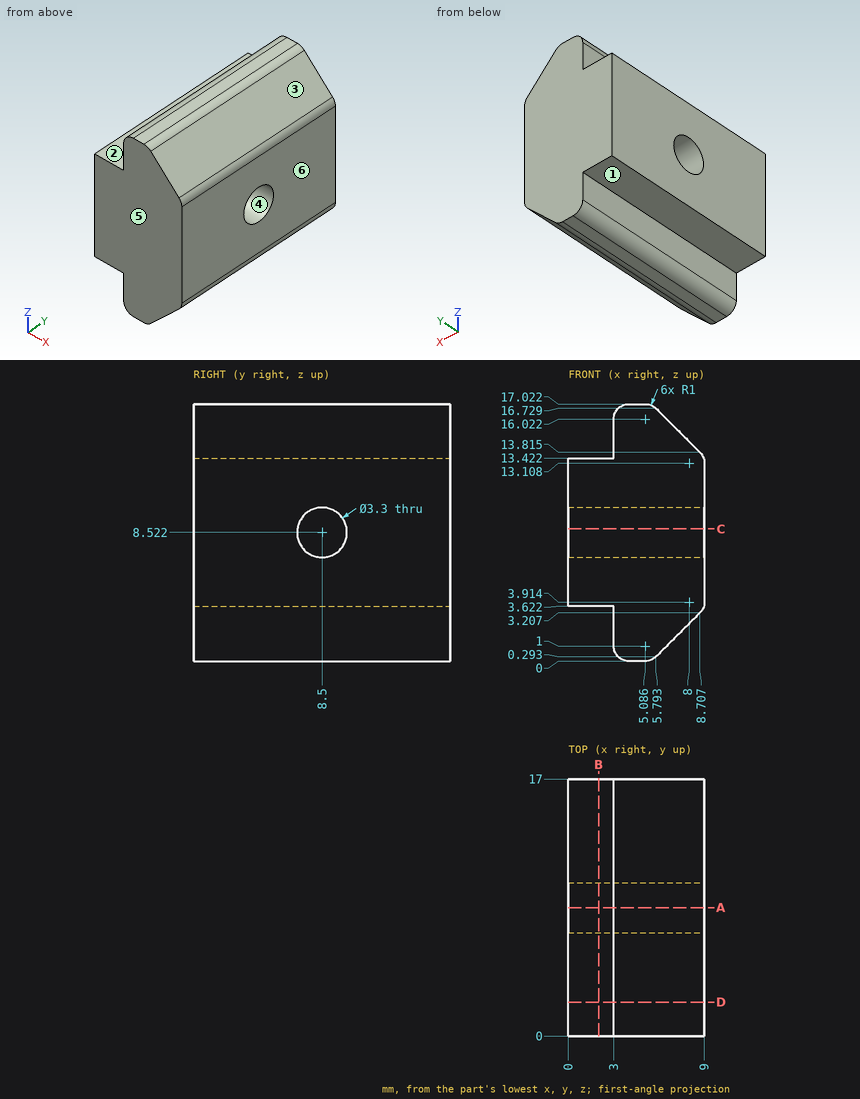
Here's the drawing with two shaded views (mm, measured from the low corner). I have some questions. A direction names the side the tool comes from. Coordinates: 2 decimals unless noted, no trailing zeros. Write each loop counter-clockwise with the first axis right and the second up, starting at its lowest first coordinate (ties: lowest second). Pieces come first, ordered by that corner, then holes. Notation, with made-up numbers: M 69.25,-19 L 116.25,-19 A13 ccw 116.25,-15 Z; hole C 20.5,51.25 d6. An arc over 180 degrees is marked long. Answer as CSV lines item,"result".
Item 1: Imagine slicing it at A-A on y = 8.5. List the corners of the cut face in (x, z) for me (1 decimal).
Geometry results:
outline,"M 0,3.6 L 3,3.6 L 3,1 A1 ccw 4,0 L 5.1,0 A1 ccw 5.8,0.3 L 8.7,3.2 A1 ccw 9,3.9 L 9,6.9 L 0,6.9 Z; M 0,10.2 L 9,10.2 L 9,13.1 A1 ccw 8.7,13.8 L 5.8,16.7 A1 ccw 5.1,17 L 4,17 A1 ccw 3,16 L 3,13.4 L 0,13.4 Z"
Item 2: I'm going to push flat-ended pins straight in: P1, Ø2, axis at y = 7, z = 2.5, coming from the -X side; P2, Ø2.5, axis at x = 1.5, y = 6, coming from the +Z side; P3, Ø0.9, axis at x = 1.5, y = 4.5, coming from the -Z side. Where does each tip first touch, or does it pass through?
Geometry results:
P1,"stops at x = 3"
P2,"stops at z = 13.42"
P3,"stops at z = 3.62"
Item 3: Imagine slicing it at D-D on y = 2.25. List the corners of the cut face in (x, z) for me (1 decimal).
Geometry results:
outline,"M 0,3.6 L 3,3.6 L 3,1 A1 ccw 4,0 L 5.1,0 A1 ccw 5.8,0.3 L 8.7,3.2 A1 ccw 9,3.9 L 9,13.1 A1 ccw 8.7,13.8 L 5.8,16.7 A1 ccw 5.1,17 L 4,17 A1 ccw 3,16 L 3,13.4 L 0,13.4 Z"
Item 4: Imagine slicing it at B-B on x = 2. List the corners of the cut face in (y, z) for me, plus the area to 3 significant figures.
Geometry results:
outline,"M 0,3.62 L 17,3.62 L 17,13.42 L 0,13.42 Z; hole C 8.5,8.52 d3.3"
area,"158 mm2"
Item 5: Please list where these lines run through material, in increasing order: line 1 along Y through (x, z) = (4, 7.5) (1 decimal); line 2 along Z through (x, y) = (6.5, 12.5); line 3 along Z through (x, y) = (1.5, 2.75).
Geometry results:
line 1,"y = 0 to 7.2, 9.8 to 17"
line 2,"z = 1 to 16.02"
line 3,"z = 3.62 to 13.42"
Item 6: We'd pull the mould along Y, two halves only. Please class the marked faces 4, 5 and 6: +Y half, -Y half, draft (parallel to the pull), parting line (faces both ways), or undercut.
Geometry results:
face 4,"undercut"
face 5,"-Y half"
face 6,"draft"
Item 7: Imagine slicing it at C-C on z = 8.75. List the corners of the cut face in (x, y) for me, plus the area to 3 significant figures.
Geometry results:
outline,"M 0,0 L 9,0 L 9,6.87 L 0,6.87 Z; M 0,10.13 L 9,10.13 L 9,17 L 0,17 Z"
area,"124 mm2"
Item 8: On a 3-axis mill with a long thin cutter (end or side, diameter ignored), from which of +Z, -Z, +X, -X, +Y, -Y can I reach the whole of each face in a straight line? I mean the marked faces 1, 2 and 3. Say none if no direction works.
Geometry results:
face 1,"-Z, -X, +Y, -Y"
face 2,"+Z, -X, +Y, -Y"
face 3,"+Z, +X, +Y, -Y"
